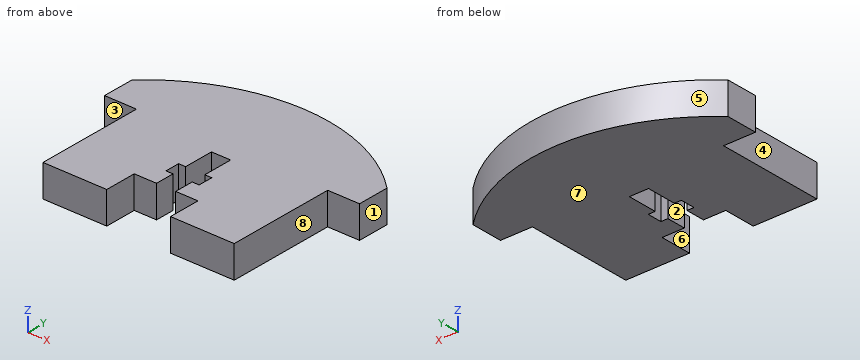
```python
from build123d import *

# Parameters (mm, degrees)
BOSS_EXTRU_1_DEPTH = 5


with BuildPart() as part:
    # Esquisse1 → Boss.-Extru.1 (new body)
    with BuildSketch(Plane.XY):
        with BuildLine():
            Line((-1.5, 3), (-1.5, 0))
            Line((-1.5, 0), (-5, 0))
            Line((-5, 0), (-5, -5))
            Line((-5, -5), (-15, -5))
            Line((-15, -5), (-15, 0))
            Line((-15, 0), (-15, 12))
            Line((-15, 12), (-20, 12))
            Line((-20, 12), (-20, 17))
            ThreePointArc((-20, 17), (0, 25), (20, 17))
            Line((20, 17), (20, 12))
            Line((20, 12), (15, 12))
            Line((15, 12), (15, 0))
            Line((15, 0), (15, -5))
            Line((15, -5), (5, -5))
            Line((5, -5), (5, 0))
            Line((5, 0), (1.5, 0))
            Line((1.5, 0), (1.5, 3))
            Line((1.5, 3), (2.6, 3))
            Line((2.6, 3), (2.6, 5.3))
            Line((2.6, 5.3), (1.5, 5.3))
            Line((1.5, 5.3), (1.5, 10))
            Line((1.5, 10), (-1.5, 10))
            Line((-1.5, 10), (-1.5, 5.3))
            Line((-1.5, 5.3), (-2.6, 5.3))
            Line((-2.6, 5.3), (-2.6, 3))
            Line((-2.6, 3), (-1.5, 3))
        make_face()
    extrude(amount=BOSS_EXTRU_1_DEPTH)


solid = part.part
```
The model under review builds one solid part; all positions refer to its coordinate system, in mm. Face numbers are marked on the shaded views. A direction names the side the tool comes from. Round coordinates to 2 decimals unless told otherwise and drop trailing zeros. Loops run counter-clockwise (first coordinate to the right, second up) from the corner with the lowest first, then second, coordinate; pieces in that order, holes last. Notation, with made-up numbers: (66, -0.5) - (119, -0.5) arc R17 ccw to (119, 22.5) - close; hole circle Ø10 at (7.5, 9.25). An arc over 180 degrees is marked (long way). Use a Markdown table: item, result. Add a question column.
Q1. Machinability: for the marked faces 4, 5, 6, 7 and 8, which of the approach directions +Z, -Z, +X, -X, +Y, -Y give a long, thin tool a straight path to every point of the face, cutting with its end or side? Answer none if there is none.
Q2. Add section A-A (y = 4). State the section outline as (x, z) points.
Q3. Add section C-C (x = -2). State the section outline as (y, z) points.
Q4. For probe 1 along X at (y, z) = (1, 3.75); probe 2 along X at (y, z) = (3.5, 4.05); probe 3 along Y at (x, z) = (-2, 0.55), list the stretches that pass through material, from the lowest coordinate up.
Q5. Add section D-D (y = 19.5). State the section outline as (x, z) points, plus the area to 3 significant figures.
Q6. The part is to be moulded in two halves that separate along X. For the marked faces 1, 2 and 3, say which applies: pulls with the +X half, pulls with the -X half, needs draft (parallel to the pull), parting line crosses it, or undercut.
Q7. Add section B-B (z = 2.95). State the section outline as (x, y) points.
Q8. Insertion check: pin 1 Ø1.8 at (y, z) = (4.5, 3) entering from -X; pin 2 Ø1 at (x, z) = (-5, 1) entering from +Y; pin 3 Ø1.8 at (x, z) = (2.5, 3.5) entering from -Y. Each pin has a flat end and moves straight along its axis. Give the tip position at first contact, or say it passes through.
Worked answers:
| question | item | result |
|---|---|---|
| 1 | face 4 | +Z, -Z, -X, -Y |
| 1 | face 5 | +Z, -Z, +Y |
| 1 | face 6 | +Z, -Z, -Y |
| 1 | face 7 | -Z, +X, -X, +Y, -Y |
| 1 | face 8 | +Z, -Z, +X, -Y |
| 2 | outline | (-15, 0) - (-2.6, 0) - (-2.6, 5) - (-15, 5) - close; (2.6, 0) - (15, 0) - (15, 5) - (2.6, 5) - close |
| 3 | outline | (0, 0) - (3, 0) - (3, 5) - (0, 5) - close; (5.3, 0) - (24.93, 0) - (24.93, 5) - (5.3, 5) - close |
| 4 | probe 1 | -15 to -1.5, 1.5 to 15 |
| 4 | probe 2 | -15 to -2.6, 2.6 to 15 |
| 4 | probe 3 | 0 to 3, 5.3 to 24.93 |
| 5 | outline | (-16.99, 0) - (16.99, 0) - (16.99, 5) - (-16.99, 5) - close |
| 5 | area | 170 mm² |
| 6 | face 1 | pulls with the +X half |
| 6 | face 2 | undercut |
| 6 | face 3 | needs draft |
| 7 | outline | (-20, 12) - (-15, 12) - (-15, -5) - (-5, -5) - (-5, 0) - (-1.5, 0) - (-1.5, 3) - (-2.6, 3) - (-2.6, 5.3) - (-1.5, 5.3) - (-1.5, 10) - (1.5, 10) - (1.5, 5.3) - (2.6, 5.3) - (2.6, 3) - (1.5, 3) - (1.5, 0) - (5, 0) - (5, -5) - (15, -5) - (15, 12) - (20, 12) - (20, 17) arc R29 ccw to (-20, 17) - close |
| 8 | pin 1 | x = -15 |
| 8 | pin 2 | y = 24.65 |
| 8 | pin 3 | y = 0 |
